Autodesk Inventor part; units mm, degrees
ref_plane "Work Plane1" through (0, 0, 15) normal (0, 0, 1) x (1, 0, 0)
ref_plane "YZ Plane" through (0, 0, 0) normal (1, 0, 0) x (0, 1, 0)
ref_plane "XZ Plane" through (0, 0, 0) normal (0, 1, 0) x (-1, 0, 0)
sketch "Sketch1" plane through (0, 0, 0) normal (0, 1, 0) x (-1, 0, 0)
  circle A0 centre (0, 0) radius 15
  dimension "d0" = 30
extrude "Extrusion1" add sketch "Sketch1" along normal blind 30
sketch "Sketch2" plane through (0, 30, 0) normal (0, 1, 0) x (1, 0, 0)
  circle A0 centre (0, 0) radius 8
  dimension "d3" = 16
extrude "Extrusion2" add sketch "Sketch2" along normal blind 4
sketch "Sketch3" plane through (0, 34, 0) normal (0, 1, 0) x (1, 0, 0)
  circle A0 centre (0, 0) radius 15
  circle A1 centre (0, 0) radius 10
  dimension "d6" = 20
extrude "Extrusion3" add sketch "Sketch3" along normal blind 140 contours A1
sketch "Sketch4" plane through (0, 174, 0) normal (0, 1, 0) x (1, 0, 0)
  circle A0 centre (0, 0) radius 10
  circle A1 centre (0, 0) radius 8
  dimension "d9" = 16
extrude "Extrusion4" add sketch "Sketch4" along normal blind 3 contours A1
sketch "Sketch5" plane through (0, 177, 0) normal (0, 1, 0) x (1, 0, 0)
  point P0 (0, 0)
sketch "Sketch6" plane through (0, 0, 0) normal (1, 0, 0) x (0, 1, 0)
  line L0 (177, -8) -> (177, 8)
  line L1 (177, 0) -> (183, 0)
  line L2 (0, 0) -> (-184.47, 0)
  line L3 (0, -15) -> (0, 15)
  line L4 (0, 0) -> (184.47, 0)
  line L5 (184.47, 0) -> (161.97, 0)
  circle A0 centre (161.97, 0) radius 22.5
  line L6 (177, 0) -> (177, 6)
  line L7 (177, 6) -> (181, 6)
  line L8 (181, 6) -> (181, 8)
  line L9 (181, 8) -> (182.9997, 8)
  dimension "d12" = 6
  dimension "d14" = 184.47
  dimension "d15" = 22.5
  dimension "d16" = 6
  dimension "d17" = 4
  dimension "d18" = 2
revolve "Revolution1" add sketch "Sketch6" angle 360 about axis through (0, 0, 0) along (0, 1, 0) contours L0 L7 L8 L9 A0 L4 L1
chamfer "Chamfer1" distance 2 angle 45 2 edges at (15, 0, 0) (15, 30, 0)
ref_plane "Work Plane1" through (0, 0, 15) normal (0, 0, 1) x (1, 0, 0)
sketch "Sketch7" plane through (0, 0, 15) normal (0, 0, 1) x (1, 0, 0)
  line L0 (0, 0) -> (0, 15)
  circle A0 centre (0, 15) radius 8.5
  dimension "d23" = 15
  dimension "d24" = 17
extrude "Extrusion5" cut sketch "Sketch7" against normal through all
thread "Thread1"
chamfer "Chamfer2" distance 1 angle 45 1 edges at (-10, 174, 0)
chamfer "Chamfer3" distance 1 angle 45 1 edges at (-10, 34, 0)
properties part number "menetesorso"
The model under review builds one solid part; all positions refer to its coordinate system, in mm. A direction names the side the tool comes from. Give positions to 0.01 mm unless a question says otherwise; leave off trailing zeros. Loops run counter-clockwise (first coordinate to the right, second up) from the corner with the lowest first, then second, coordinate; pieces in that order, holes last. Notation, with made-up numbers: (4.25, -2.5) -> (29.25, -2.5) arc R21 ccw to (29.25, 10.5) -> close; hole circle Ø4 at (69, 81.5). An arc over 180 degrees is marked (long way). Answer as a JSON object with one key per item and string values. Group by question number.
Q1. Draft analysis for pull direction X (two halves, no side actions). For faces 1 (the cylindrical face through (-2.17, 103.03, -9.76)), 2 (the cylindrical face through (-6.265, 20.745, 0.21)), 3 (the flat face through (-2, 177, -6)), state which applies: pulls with the +X half, pulls with the -X half, needs draft (parallel to the pull), parting line crosses it, or undercut.
Q2. Take a section at B-B (y = 15). Write out the cut boundary in (x, z).
Q3. Tool access review of faces 4 (the conical face through (9.674, 0.125, 8.871)), 5 (the flat face through (-6, 30, 6)), 6 (the cylindrical face through (-7.81, 182.01, -1.73)): name each direction out of +Z, -Z, +X, -X, +Y, -Y from which nothing blocks a thin tool from reaching the whole face with its end or side.
Q4. Take a section at C-C (y = 37.5). Write out the cut boundary in (x, z).
Q5. Insertion check: pin 1 (6 mm diameter, centred on y = 91, z = 10.5, fed in from -X); pin 2 (5 mm diameter, centred on x = -4.5, y = 130.5, fed in from +Z); pin 3 (5 mm diameter, centred on x = 4, y = 130.5, fed in from +Z). Each pin has a flat end and moves straight along its axis. Give the tip position at first contact, or say it passes through.
Q6. Wall thickness on line 1 along Y through (x, z) = (1, 7); line 2 along Y through (x, z) = (-2, 9); line 3 along Y through (x, z) = (0, 0): over which ranges is each line inside the solid? List them lowest first.
Answer below:
{
 "1": {"face 1": "parting line crosses it", "face 2": "undercut", "face 3": "needs draft"},
 "2": {"outline": "(-8.5, -12.36) -> (-8.5, 12.36) arc R15 ccw to start; (8.5, -12.36) arc R15 ccw to (8.5, 12.36) -> close"},
 "3": {"face 4": "-Y", "face 5": "none", "face 6": "+Y"},
 "4": {"outline": "circle Ø20 at (0, 0)"},
 "5": {"pin 1": "stops at x = -6.61", "pin 2": "stops at z = 9.8", "pin 3": "stops at z = 9.89"},
 "6": {"line 1": "y = 0 to 6.56, 23.44 to 177, 181 to 183.33", "line 2": "y = 0 to 6.74, 23.26 to 30, 34.22 to 173.78", "line 3": "y = 0 to 6.5, 23.5 to 184.47"}
}
